Can you work these out from the model? Positions are in its coordinate system, mm. Face numbers are marked on the shaded views. A direction names the side the tool comes from. Give positions to 0.01 mm unless a question says otherwise; leave off trailing zeros. Loops run counter-clockwise (first coordinate to the right, second up) from the corner with the lowest first, then second, coordinate; pieces in that order, holes last. Notation, with made-up numbers: (61.5, -16.75) - (116.5, -16.75) arc R9 ccw to (116.5, -4.75) - close; hole circle Ø5 at (84, 59.25). An arc over 180 degrees is marked (long way). Write item = value, one per line.
from build123d import *

# Parameters (mm, degrees)
F0_W     = 360
F0_H     = 500
F1_DEPTH = 15
F2_W     = 150
F2_H     = 500
F3_DEPTH = 15
F5_D     = 5
F5_DEPTH = 5
F5_TIP   = 1.5021515476


with BuildPart() as f1:
    # F0 (on Front) → F1 (new body)
    with BuildSketch(Plane.XZ):
        with Locations((-21.0021212956, 2.1194461733)):
            Rectangle(F0_W, F0_H)
    extrude(amount=-F1_DEPTH)

    # F2 (on face) → F3 (join)
    with BuildSketch(Plane(origin=(0, 15, 0), x_dir=(-1, 0, 0), z_dir=(0, 1, 0))):
        with Locations((34.7477533389, 2.1194461733)):
            Rectangle(F2_W, F2_H)
    extrude(amount=F3_DEPTH)

    # F5
    with Locations(Plane(origin=(0, 30, 0), x_dir=(-1, 0, 0), z_dir=(0, 1, 0))):
        with Locations((-28.9978787044, 92.1194461733), (71.0021212956, 92.1194461733), (71.0021212956, -7.8805538267), (-28.9978787044, -7.8805538267)):
            Hole(F5_D / 2, depth=F5_DEPTH)
            with Locations((0, 0, -(F5_DEPTH + F5_TIP / 2))):  # 118° drill point
                Cone(0, F5_D / 2, F5_TIP, mode=Mode.SUBTRACT)


solid = f1.part
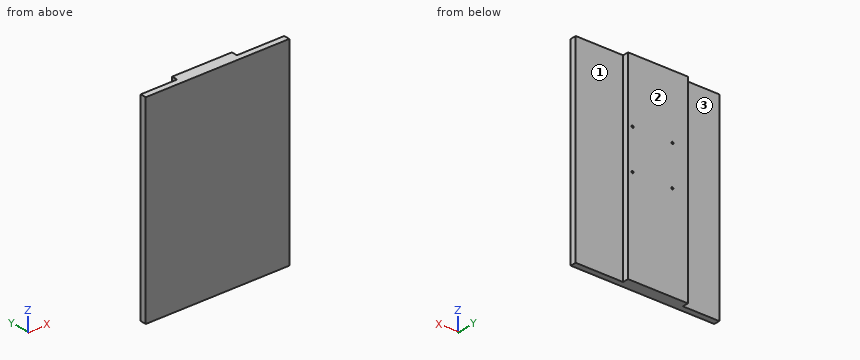
Q1. I need wall thicknesses on L1, parallel to X at y = 27.25, z = -168; L2, parallel to Y at x = 101, z = 217. Which ranges of each line are inside material? Lowest first, please.
Output:
L1 = -109.75 to 40.25
L2 = 0 to 15
Q2. For pin 1 (16.5 mm diameter, centred on y = 25.5, z = 63.5, fed in from -X); pin 2 (7.5 mm diameter, centred on y = 25.5, z = -75.5, fed in from +X); pin 3 (1 mm diameter, centred on x = -155, z = -97, fed in from +Y), each with a flat end and sliding along its axis, tell me the tip position at first contact or that it passes through.
Output:
pin_1 = -109.75
pin_2 = 40.25
pin_3 = 15
Q3. Imagine slicing it at B-B, the plane x = 86.5. Write out the boundary of the cut face in (y, z).
Output:
outline = (0, -247.88) - (15, -247.88) - (15, 252.12) - (0, 252.12) - close
Q4. Imagine slicing it at A-A, the plane z = -138.5. Write out the boundary of the cut face in (x, y), then the cut area to 3 significant figures.
Output:
outline = (-201, 0) - (159, 0) - (159, 15) - (40.25, 15) - (40.25, 30) - (-109.75, 30) - (-109.75, 15) - (-201, 15) - close
area = 7,650 mm2
Q5. Which directions (+Z, -Z, +X, -X, +Y, -Y) give clear straight access to the entire face, cutting with the end or side of a thin tool? Please do the marked faces 1, 2 and 3.
Output:
face_1 = +Z, -Z, +X, +Y
face_2 = +Z, -Z, +X, -X, +Y
face_3 = +Z, -Z, -X, +Y
